Can you work these out from the model? Positions are in its coordinate system, mm. Face numbers are marked on the shaded views. A direction names the side the tool comes from. Give positions to 0.01 mm unless a question says otherwise; leave off trailing zeros. Order: outer loops, then holes, each group sorted by start corner. A loop starts at its lowest first (then second) coordinate and runs counter-clockwise, first axis right, second up. Notation, with made-up numbers: (-13.75, 74) - (5.25, 74) arc R19 cw to (5.25, 110) - close; hole circle Ø1 at (45, 31.25). An arc over 180 degrees is marked (long way). One line per question, with ' | ' between items.
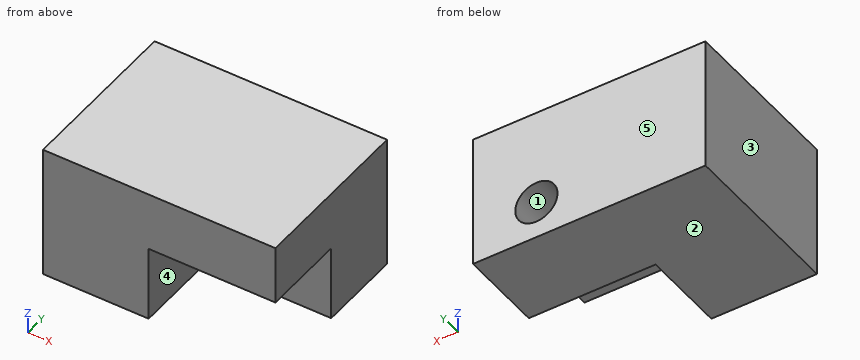
```python
from build123d import *

# Parameters (mm, degrees)
F0_W     = 55
F0_H     = 32
F1_DEPTH = 40
F2_W     = 30
F2_H     = 18
F3_DEPTH = 20
F4_R     = 5
F5_DEPTH = 20.001


with BuildPart() as f1:
    # F0 (on Front) → F1 (new body)
    with BuildSketch(Plane.XZ):
        with Locations((27.5, -16)):
            Rectangle(F0_W, F0_H)
    extrude(amount=F1_DEPTH)

    # F2 (on face) → F3 (cut)
    with BuildSketch(Plane.XZ.offset(40)):
        with Locations((40, -23)):
            Rectangle(F2_W, F2_H)
    extrude(amount=-F3_DEPTH, mode=Mode.SUBTRACT)

    # F4 (on face) → F5 (cut, through all)
    with BuildSketch(Plane.XZ.offset(20)):
        with Locations((40, -23)):
            Circle(F4_R)
    extrude(amount=-F5_DEPTH, mode=Mode.SUBTRACT)


solid = f1.part
```
(1) Imagine slicing it at A-A (z = -23). List the corners of the cut face in (x, y) for me.
Answer below:
outline: (0, -40) - (25, -40) - (25, -20) - (35, -20) - (35, 0) - (0, 0) - close; (45, -20) - (55, -20) - (55, 0) - (45, 0) - close
(2) Imagine slicing it at D-D (y = -14.5). List the corners of the cut face in (x, z) for me, and give its area (3 significant figures).
Answer below:
outline: (0, -32) - (55, -32) - (55, 0) - (0, 0) - close; hole circle Ø10 at (40, -23) | area: 1,680 mm^2
(3) If I drill on line 1 (Z direction, x = 40, y = -12); line 2 (X direction, y = -23.5, z = -18); line 3 (X direction, y = -19.5, z = -24.5), over which ranges is the centre line in solid material (lowest first)?
Answer below:
line 1: -32 to -28, -18 to 0 | line 2: 0 to 25 | line 3: 0 to 35.23, 44.77 to 55
(4) Imagine slicing it at C-C (y = -26). List the corners of the cut face in (x, z) for me, and give its area (3 significant figures).
Answer below:
outline: (0, -32) - (25, -32) - (25, -14) - (55, -14) - (55, 0) - (0, 0) - close | area: 1,220 mm^2
(5) Imagine slicing it at B-B (x = 43). List the corners of the cut face in (y, z) for me.
Answer below:
outline: (-40, -14) - (-20, -14) - (-20, -19) - (0, -19) - (0, 0) - (-40, 0) - close; (-20, -32) - (0, -32) - (0, -27) - (-20, -27) - close
(6) Will these pins go through, and if not, where does the flat tip stop? pin 1 (1.5 mm diameter, centred on y = -29, z = -17.5, fed in from +X); pin 2 (10 mm diameter, centred on x = 47.5, y = -35.5, fed in from -Z); pin 3 (11.5 mm diameter, centred on x = 40, z = -23, fed in from -Y).
Answer below:
pin 1: x = 25 | pin 2: z = -14 | pin 3: y = -20
(7) If we mould it in two halves opening along Z, with no side actions, what happens to the marked faces 1, 2 and 3? For each: released by +Z, released by -Z, zero draft, split by the parting line, or undercut.
Answer below:
face 1: undercut | face 2: released by -Z | face 3: zero draft
(8) On a 3-axis mill with a long thin cutter (end or side, diameter ignored), from which of +Z, -Z, +X, -X, +Y, -Y can I reach the whole of each face in a straight line? I mean the marked faces 4 and 5. Say none if no direction works.
Answer below:
face 4: -Z, +X, -Y | face 5: +Z, -Z, +X, -X, +Y
